from build123d import *

# Parameters (mm, degrees)
SKETCH1_R           = 16.5
SKETCH1_R_2         = 2
BOSS_EXTRUDE3_DEPTH = 10
SKETCH2_R           = 19.5
CUT_EXTRUDE1_DEPTH  = 10
CUT_EXTRUDE2_DEPTH  = 10
CUT_EXTRUDE3_DEPTH  = 10
CUT_EXTRUDE6_DEPTH  = 10
SKETCH9_W           = 90
SKETCH9_H           = 10
BOSS_EXTRUDE4_DEPTH = 15
FILLET1_R           = 5
SKETCH10_R          = 4.25
CUT_EXTRUDE7_DEPTH  = 10
CUT_EXTRUDE8_DEPTH  = 10


with BuildPart() as part:
    # Sketch1 → Boss-Extrude3 (new body)
    with BuildSketch(Plane(origin=(0, 0, 0), x_dir=(1, 0, 0), z_dir=(0, 1, 0))):
        with BuildLine():
            Line((-52.326392464, -141.880675109), (47.673607536, -141.880675109))
            Line((47.673607536, -141.880675109), (47.673607536, 8.119324891))
            ThreePointArc((47.673607536, 8.119324891), (-2.326392464, 58.119324891), (-52.326392464, 8.119324891))
            Line((-52.326392464, 8.119324891), (-52.326392464, -141.880675109))
        make_face()
        with Locations((-2.326392464, 8.119324891)):
            Circle(SKETCH1_R, mode=Mode.SUBTRACT)
        with Locations((21.173607536, 8.119324891)):
            Circle(SKETCH1_R_2, mode=Mode.SUBTRACT)
        with Locations((9.423607536, -12.232272098)):
            Circle(SKETCH1_R_2, mode=Mode.SUBTRACT)
        with Locations((-14.076392464, -12.232272098)):
            Circle(SKETCH1_R_2, mode=Mode.SUBTRACT)
        with Locations((-25.826392464, 8.119324891)):
            Circle(SKETCH1_R_2, mode=Mode.SUBTRACT)
        with Locations((-14.076392464, 28.47092188)):
            Circle(SKETCH1_R_2, mode=Mode.SUBTRACT)
        with Locations((9.423607536, 28.47092188)):
            Circle(SKETCH1_R_2, mode=Mode.SUBTRACT)
        with Locations((-47.326392464, -116.880675109)):
            Circle(SKETCH1_R_2, mode=Mode.SUBTRACT)
        with Locations((42.673607536, -116.880675109)):
            Circle(SKETCH1_R_2, mode=Mode.SUBTRACT)
        with Locations((-37.326392464, -126.880675109)):
            Circle(SKETCH1_R_2, mode=Mode.SUBTRACT)
        with Locations((-37.326392464, -96.880675109)):
            Circle(SKETCH1_R_2, mode=Mode.SUBTRACT)
        with Locations((-47.326392464, -76.880675109)):
            Circle(SKETCH1_R_2, mode=Mode.SUBTRACT)
        with Locations((42.673607536, -76.880675109)):
            Circle(SKETCH1_R_2, mode=Mode.SUBTRACT)
        with Locations((-47.326392464, -56.880675109)):
            Circle(SKETCH1_R_2, mode=Mode.SUBTRACT)
        with Locations((42.673607536, -56.880675109)):
            Circle(SKETCH1_R_2, mode=Mode.SUBTRACT)
        with Locations((-27.326392464, -116.880675109)):
            Circle(SKETCH1_R_2, mode=Mode.SUBTRACT)
        with Locations((22.673607536, -116.880675109)):
            Circle(SKETCH1_R_2, mode=Mode.SUBTRACT)
        with Locations((-27.326392464, -56.880675109)):
            Circle(SKETCH1_R_2, mode=Mode.SUBTRACT)
        with Locations((-27.326392464, -76.880675109)):
            Circle(SKETCH1_R_2, mode=Mode.SUBTRACT)
        with Locations((22.673607536, -56.880675109)):
            Circle(SKETCH1_R_2, mode=Mode.SUBTRACT)
        with Locations((22.673607536, -76.880675109)):
            Circle(SKETCH1_R_2, mode=Mode.SUBTRACT)
        with Locations((32.673607536, -96.880675109)):
            Circle(SKETCH1_R_2, mode=Mode.SUBTRACT)
        with Locations((32.673607536, -126.880675109)):
            Circle(SKETCH1_R_2, mode=Mode.SUBTRACT)
    extrude(amount=BOSS_EXTRUDE3_DEPTH)

    # Sketch2 → Cut-Extrude1 (cut)
    with BuildSketch(Plane(origin=(0, 10, 0), x_dir=(1, 0, 0), z_dir=(0, 1, 0))):
        with Locations((-2.326392464, -96.880675109)):
            Circle(SKETCH2_R)
    extrude(amount=-CUT_EXTRUDE1_DEPTH, mode=Mode.SUBTRACT)

    # Sketch3 → Cut-Extrude2 (cut)
    with BuildSketch(Plane(origin=(0, 10, 0), x_dir=(1, 0, 0), z_dir=(0, 1, 0))):
        with BuildLine():
            Line((-7.326392464, -131.880675109), (-7.326392464, -115.728751934))
            ThreePointArc((-7.326392464, -115.728751934), (-2.326392464, -116.380675109), (2.673607536, -115.728751934))
            Line((2.673607536, -115.728751934), (2.673607536, -131.880675109))
            Line((2.673607536, -131.880675109), (-7.326392464, -131.880675109))
        make_face()
    extrude(amount=-CUT_EXTRUDE2_DEPTH, mode=Mode.SUBTRACT)

    # Sketch4 → Cut-Extrude3 (cut)
    with BuildSketch(Plane(origin=(0, 10, 0), x_dir=(1, 0, 0), z_dir=(0, 1, 0))):
        with BuildLine():
            ThreePointArc((-19.688674915, -88.003674033), (-16.114974697, -83.092092876), (-11.203393541, -79.518392659))
            Line((-11.203393541, -79.518392659), (-16.114974697, -74.606811502))
            Line((-16.114974697, -74.606811502), (-24.600256072, -83.092092876))
            Line((-24.600256072, -83.092092876), (-19.688674915, -88.003674033))
        make_face()
        with BuildLine():
            Line((11.462189769, -74.606811502), (6.550608612, -79.518392659))
            ThreePointArc((6.550608612, -79.518392659), (11.462189769, -83.092092876), (15.035889986, -88.003674033))
            Line((15.035889986, -88.003674033), (19.947471143, -83.092092876))
            Line((19.947471143, -83.092092876), (11.462189769, -74.606811502))
        make_face()
        with BuildLine():
            Line((19.947471143, -110.669257342), (15.035889986, -105.757676186))
            ThreePointArc((15.035889986, -105.757676186), (11.462189769, -110.669257342), (6.550608612, -114.24295756))
            Line((6.550608612, -114.24295756), (11.462189769, -119.154538717))
            Line((11.462189769, -119.154538717), (19.947471143, -110.669257342))
        make_face()
        with BuildLine():
            ThreePointArc((-11.203393541, -114.24295756), (-16.114974697, -110.669257342), (-19.688674915, -105.757676186))
            Line((-19.688674915, -105.757676186), (-24.600256072, -110.669257342))
            Line((-24.600256072, -110.669257342), (-16.114974697, -119.154538717))
            Line((-16.114974697, -119.154538717), (-11.203393541, -114.24295756))
        make_face()
    extrude(amount=-CUT_EXTRUDE3_DEPTH, mode=Mode.SUBTRACT)

    # Sketch8 → Cut-Extrude6 (cut)
    with BuildSketch(Plane(origin=(0, 10, 0), x_dir=(1, 0, 0), z_dir=(0, 1, 0))):
        with BuildLine():
            Line((-21.826392464, -96.880675109), (17.173607536, -96.880675109))
            Line((17.173607536, -96.880675109), (17.173607536, -72.880675109))
            ThreePointArc((17.173607536, -72.880675109), (-2.326392464, -53.380675109), (-21.826392464, -72.880675109))
            Line((-21.826392464, -72.880675109), (-21.826392464, -96.880675109))
        make_face()
    extrude(amount=-CUT_EXTRUDE6_DEPTH, mode=Mode.SUBTRACT)

    # Sketch9 → Boss-Extrude4 (add)
    with BuildSketch(Plane.ZY.offset(52.326392464)):
        with Locations((96.880675109, 5)):
            Rectangle(SKETCH9_W, SKETCH9_H)
    extrude(amount=BOSS_EXTRUDE4_DEPTH)

    # Fillet1
    fillet1_edges = [part.edges().sort_by_distance(p)[0] for p in [
        (-67.326392464, 5, 51.880675109),
    ]]
    fillet(fillet1_edges, radius=FILLET1_R)

    # Sketch10 → Cut-Extrude7 (cut)
    with BuildSketch(Plane(origin=(0, 10, 0), x_dir=(1, 0, 0), z_dir=(0, 1, 0))):
        with Locations((-56.326392464, -65.880675109)):
            Circle(SKETCH10_R)
    extrude(amount=-CUT_EXTRUDE7_DEPTH, mode=Mode.SUBTRACT)

    # Sketch11 → Cut-Extrude8 (cut)
    with BuildSketch(Plane(origin=(0, 10, 0), x_dir=(1, 0, 0), z_dir=(0, 1, 0))):
        with BuildLine():
            Line((15.673607536, -42.630675109), (33.673607536, -42.630675109))
            ThreePointArc((33.673607536, -42.630675109), (37.923607536, -46.880675109), (33.673607536, -51.130675109))
            Line((33.673607536, -51.130675109), (15.673607536, -51.130675109))
            ThreePointArc((15.673607536, -51.130675109), (11.423607536, -46.880675109), (15.673607536, -42.630675109))
        make_face()
        with BuildLine():
            Line((-38.326392464, -42.630675109), (-20.326392464, -42.630675109))
            ThreePointArc((-20.326392464, -42.630675109), (-16.076392464, -46.880675109), (-20.326392464, -51.130675109))
            Line((-20.326392464, -51.130675109), (-38.326392464, -51.130675109))
            ThreePointArc((-38.326392464, -51.130675109), (-42.576392464, -46.880675109), (-38.326392464, -42.630675109))
        make_face()
    extrude(amount=-CUT_EXTRUDE8_DEPTH, mode=Mode.SUBTRACT)


solid = part.part
Geometry check sheet. Reference: the model listing, model coordinates, mm. Coordinates: 2 decimals unless noted, no trailing zeros. Loops run counter-clockwise (first coordinate to the right, second up) from the corner with the lowest first, then second, coordinate; pieces in that order, holes last. Notation, with made-up numbers: (-19.5, 71) - (3.5, 71) arc R28 cw to (3.5, 100) - close; hole circle Ø9 at (-12, -22). An arc over 180 degrees is marked (long way). Use one line per item in the form item = value. Start each with the question number.
Item 1: Section check C-C, the plane z = 23.5. Enter the section's corners in (x, y).
Item 2: Section check D-D, the plane y = 3.5. Give the number of separate pieces and of enclosed holes in the cut face, and give its area (3 significant figures).
Item 3: Thickness scan on probe 1 along X at (y, z) = (9, 12.5); probe 2 along Z at (x, y) = (-16.5, 4.5); probe 3 along Z at (x, y) = (-25, 9). Record the ranges inside material, lowest first.
Item 4: Section check A-A, the plane z = -4. Enter the section's corners in (x, y), and give its area (3 significant figures).
Item 5: Section check B-B, the plane x = 0.5. Enter the section's corners in (y, z).
Item 6: Mould release check, pull along Z, two halves, no side actions. Record for faces 1 (the face through (-56.88, 5.07, 61.667)), 2 (the face through (-1.227, 4.93, -58.107)), 3 (the face through (47.674, 5, 68)): +Z half, -Z half, draft (parallel to the pull), parting line (faces both ways), or undercut.
Item 7: Gauge pin test, flat ends, axial feed: pin 1 (4.5 mm diameter, centred on x = -37.33, z = 96.88, fed in from -Y); pin 2 (5 mm diameter, centred on x = 22, y = 3, fed in from -Z); pin 3 (3 mm diameter, centred on x = 23, y = 5, fed in from -Z). Record the tip position at first contact, or that the pin passes through.
Computed:
q1.outline = (-52.33, 0) - (47.67, 0) - (47.67, 10) - (-52.33, 10) - close
q2.separate_pieces = 1
q2.enclosed_holes = 27
q2.area = 16,200 mm2
q3.probe_1 = -52.33 to -16.06, -12.09 to 7.44, 11.41 to 47.67
q3.probe_2 = -56.07 to -16.57, 0.33 to 45.03, 48.73 to 59.49, 118.77 to 141.88
q3.probe_3 = -52.68 to -9.94, -6.3 to 42.63, 51.13 to 141.88
q4.outline = (-52.33, 0) - (-18.3, 0) - (-18.3, 10) - (-52.33, 10) - close; (13.65, 0) - (47.67, 0) - (47.67, 10) - (13.65, 10) - close
q4.area = 680 mm2
q5.outline = (0, -58.04) - (10, -58.04) - (10, -24.38) - (0, -24.38) - close; (0, 8.14) - (10, 8.14) - (10, 53.59) - (0, 53.59) - close; (0, 131.88) - (10, 131.88) - (10, 141.88) - (0, 141.88) - close
q6.face_1 = undercut
q6.face_2 = -Z half
q6.face_3 = draft
q7.pin_1 = 0
q7.pin_2 = -53.1
q7.pin_3 = -52.08
